Autodesk Inventor part; units mm, degrees
ref_plane "YZ Plane" through (0, 0, 0) normal (1, 0, 0) x (0, 1, 0)
ref_plane "XZ Plane" through (0, 0, 0) normal (0, 1, 0) x (-1, 0, 0)
ref_plane "XY Plane" through (0, 0, 0) normal (0, 0, 1) x (1, 0, 0)
sketch "Sketch1" plane through (0, 0, 0) normal (1, 0, 0) x (0, 1, 0)
  line L0 (0, 0) -> (0, -127)
  line L1 (0, -127) -> (50.8, -127)
  line L2 (0, 0) -> (50.8, -127)
  dimension "d0" = 127
  dimension "d1" = 50.8
extrude "Extrusion1" add sketch "Sketch1" along normal blind 101.6
shell "Shell1" thickness 2.54 removed faces 1 at (33.8667, 33.8667, -84.6667)
sketch "Sketch2" plane through (0, 0, -127) normal (0, -1, 0) x (1, 0, 0)
  line L0 (0, 127) -> (0, 0)
  line L1 (0, 0) -> (101.6, 0)
  line L2 (101.6, 127) -> (101.6, 0)
  line L3 (0, 127) -> (101.6, 127)
  point P0 (25.4, 30.48)
  point P1 (25.4, 74.93)
  point P2 (76.2, 74.93)
  point P3 (76.2, 30.48)
  dimension "d5" = 30.48
  dimension "d6" = 30.48
  dimension "d7" = 25.4
  dimension "d8" = 25.4
  dimension "d9" = 25.4
  dimension "d10" = 25.4
  dimension "d11" = 44.45
  dimension "d12" = 44.45
hole "Hole1" at (25.4, 0, -96.52) at (25.4, 0, -52.07) at (76.2, 0, -52.07) at (76.2, 0, -96.52) direction (0, 1, 0) diameter 8 depth 19.05 tip angle 118
properties part number "Bucket" material "Aluminum 6061"
Design review of the part built by this model. Coordinates are the model's own, in mm. A direction names the side the tool comes from. Coordinates: 2 decimals unless noted, no trailing zeros. Loops run counter-clockwise (first coordinate to the right, second up) from the corner with the lowest first, then second, coordinate; pieces in that order, holes last.
Item 1: For faces 5 (the flat face through (99.06, 15, -91)), 6 (the flat face through (50.563, 0.822, -2.056)), list the 3-axis set-ups (+Z, -Z, +X, -X, +Y, -Y) from which the entire face can be reached by the end or side of a thin tool; tool diameter is ignored.
Completed:
face 5: +Z, +Y
face 6: +Z, +X, -X, +Y
Item 2: Add section A-A (x = 25.4). Write out the cut boundary in (y, z), and give its area (3 significant figures).
Completed:
outline: (0, -127) - (50.8, -127) - (49.78, -124.46) - (2.54, -124.46) - (2.54, -100.52) - (0, -100.52) - close; (0, -92.52) - (2.54, -92.52) - (2.54, -56.07) - (0, -56.07) - close; (0, -48.07) - (2.54, -48.07) - (2.54, -6.35) - (0, 0) - close
area: 395 mm2
Item 3: Draft analysis for pull direction X (two halves, no side actions). For faces 1 (the cylindrical face through (78.634, 1.288, -48.896)), 2 (the flat face through (0, 14, -91)), 3 (the flat face through (50, 26, -124.46)), 4 (the flat face through (50, 25, -127)), state which applies: pulls with the +X half, pulls with the -X half, needs draft (parallel to the pull), parting line crosses it, or undercut.
Completed:
face 1: undercut
face 2: pulls with the -X half
face 3: undercut
face 4: needs draft
Item 4: Add section D-D (z = -75). Write out the cut boundary in (x, y), and give its area (3 significant figures).
Completed:
outline: (0, 0) - (101.6, 0) - (101.6, 30) - (99.06, 30) - (99.06, 2.54) - (2.54, 2.54) - (2.54, 30) - (0, 30) - close
area: 398 mm2
Item 5: Wall thickness on L1, parallel to X at y = 1.85, z = -96.52; L2, parallel to X at y = 13.5, z = -85.5; L3, parallel to Z at x = 25.4, y = 0.5: over which ranges is each line inside the solid? List them lowest first.
Completed:
L1: x = 0 to 21.4, 29.4 to 72.2, 80.2 to 101.6
L2: x = 0 to 2.54, 99.06 to 101.6
L3: z = -127 to -100.52, -92.52 to -56.07, -48.07 to -1.25
Item 6: Clearance check with flat-ended pins moving along their axes: pin 1 (10 mm diameter, centred on x = 53.5, y = 33.5, fed in from +Z); pin 2 (10 mm diameter, centred on x = 44.5, z = -102.5, fed in from +Y). State where each tip first meets the part, or that it passes through.
Completed:
pin 1: stops at z = -124.46
pin 2: stops at y = 2.54
Item 7: Add section C-C (y = 19). Write out the cut boundary in (x, z).
Completed:
outline: (0, -127) - (101.6, -127) - (101.6, -47.5) - (99.06, -47.5) - (99.06, -124.46) - (2.54, -124.46) - (2.54, -47.5) - (0, -47.5) - close
Item 8: Add section B-B (z = -98). Write out the cut boundary in (x, y).
Completed:
outline: (0, 0) - (21.68, 0) - (21.68, 2.54) - (2.54, 2.54) - (2.54, 39.2) - (0, 39.2) - close; (29.12, 0) - (72.48, 0) - (72.48, 2.54) - (29.12, 2.54) - close; (79.92, 0) - (101.6, 0) - (101.6, 39.2) - (99.06, 39.2) - (99.06, 2.54) - (79.92, 2.54) - close
